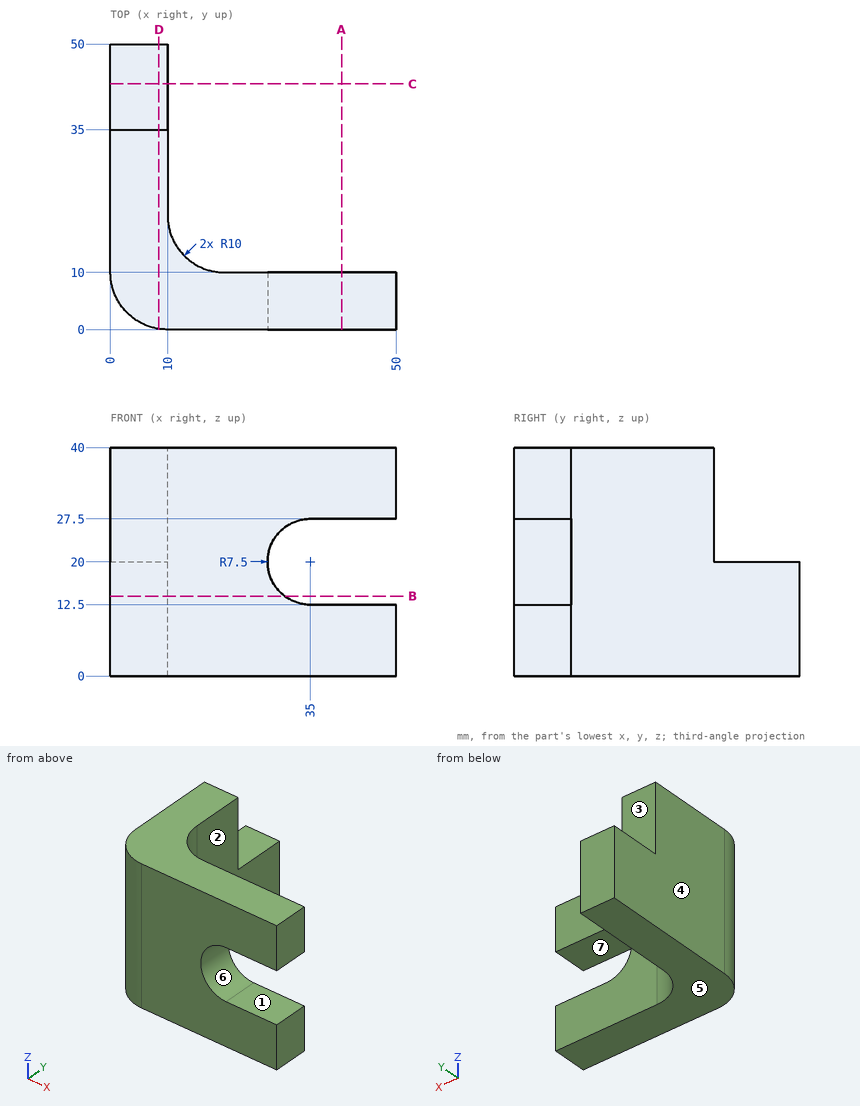
The figure shows three views and two pictorial views of one solid part (mm, origin at its lowest corner). Answer the questions. A direction names the side the tool comes from. Round coordinates to 2 decimals unless told otherwise and drop trailing zeros. Loops run counter-clockwise (first coordinate to the right, second up) from the corner with the lowest first, then second, coordinate; pieces in that order, holes last. Notation, with made-up numbers: (-27.75, 45.25) -> (-14.75, 45.25) arc R12 ccw to (-14.75, 64.25) -> close; hole circle Ø2 at (-25.75, 87.5). An arc over 180 degrees is marked (long way). Use one line per item in the form item = value.
(1) Find section D-D on x = 8.5. Give the vertices of the cut face in (y, z).
Answer list:
outline = (0.11, 0) -> (50, 0) -> (50, 20) -> (35, 20) -> (35, 40) -> (0.11, 40) -> close
(2) Straight lines are drawn through the part: line 1 (Y direction, x = 32, z = 8); line 2 (Y direction, x = 5, z = 23). For each, find the intervals that lie inside material, in ascending order.
Answer list:
line_1 = 0 to 10
line_2 = 1.34 to 35
(3) For a pull along Z with two mould halves and no side action, classify the marked faces 4, 5, 6 and 7 as released by +Z, released by -Z, zero draft, split by the parting line, or undercut.
Answer list:
face_4 = zero draft
face_5 = released by -Z
face_6 = undercut
face_7 = undercut
(4) A tool of negligible diameter and unlimited length cuts with its end or side. For the marked faces 1, 2 and 3, from which of +Z, -Z, +X, -X, +Y, -Y can it reach the whole face along a straight path? Write none if from no direction.
Answer list:
face_1 = +X, +Y, -Y
face_2 = +Z, -Z, +X, +Y
face_3 = +Z, +X, -X, +Y
(5) Find section B-B on z = 14. Give the vertices of the cut face in (x, y).
Answer list:
outline = (0, 10) arc R10 ccw to (10, 0) -> (30.5, 0) -> (30.5, 10) -> (20, 10) arc R10 cw to (10, 20) -> (10, 50) -> (0, 50) -> close
(6) Find section A-A on x = 40.5. Give the vertices of the cut face in (y, z), then the cut area to 3 significant figures.
Answer list:
outline = (0, 0) -> (10, 0) -> (10, 12.5) -> (0, 12.5) -> close; (0, 27.5) -> (10, 27.5) -> (10, 40) -> (0, 40) -> close
area = 250 mm2
(7) Find section C-C on y = 43. Give the vertices of the cut face in (x, z), then the cut area to 3 significant figures.
Answer list:
outline = (0, 0) -> (10, 0) -> (10, 20) -> (0, 20) -> close
area = 200 mm2
(8) Flat-ended cylindrical pins translate along their axes: P1, Ø15, axis at x = 31.5, z = 12.5, coming from the +Y side; P2, Ø1, axis at y = 21.5, z = 35, coming from the +X side; P3, Ø3, axis at x = 6.5, z = 29.5, coming from the +Y side. Find the tip coordinate at first contact, or state that the pin passes through.
Answer list:
P1 = 10
P2 = 10
P3 = 35
